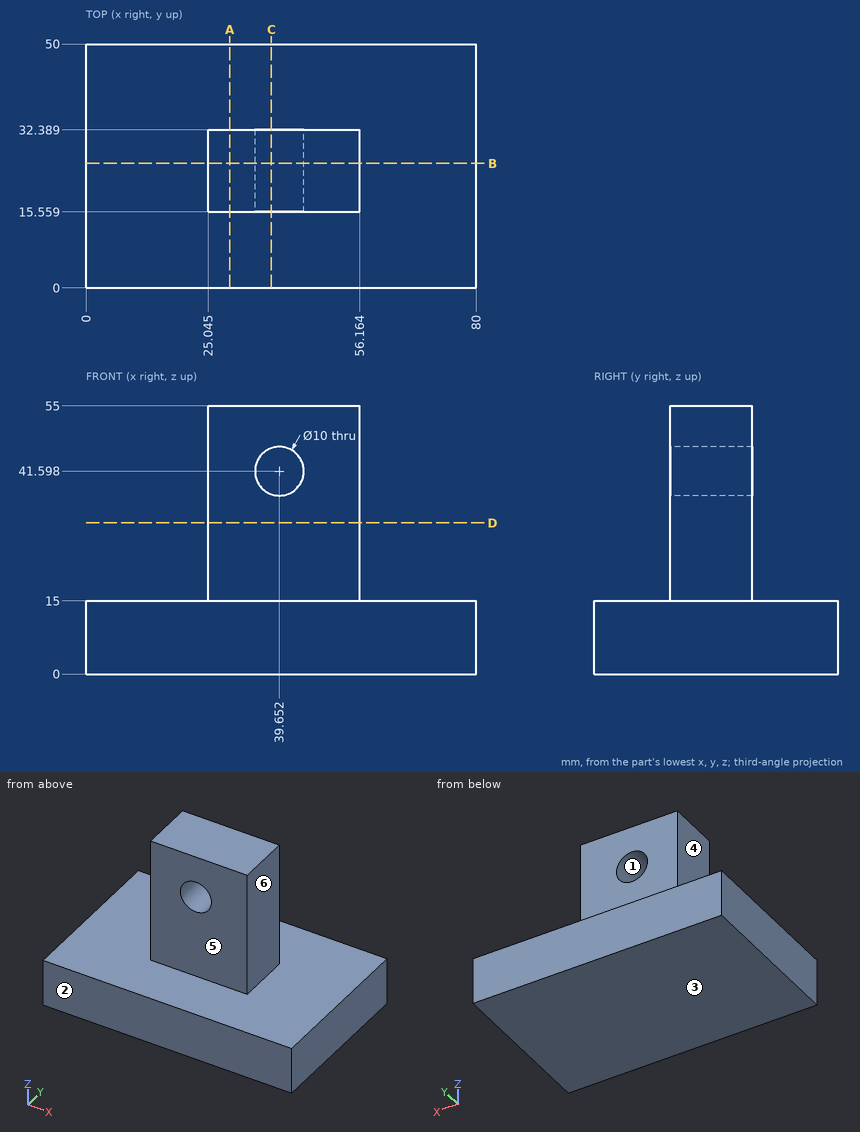
Drawing for the job (mm, zero at the part's lowest x, y, z). A direction names the side the tool comes from. Give positions to 0.01 mm unless a question says otherwise; leave off trailing zeros. Loops run counter-clockwise (first coordinate to the right, second up) from the corner with the lowest first, then second, coordinate; pieces in that order, holes last.
1) Drop flat-ended pins along their axis: P1, Ø1, axis at x = 66.5, y = 8.5, coming from the +Z side; P2, Ø9.5, axis at x = 34, z = 41, coming from the -Y side; P3, Ø6, axis at y = 13.5, z = 44.5, coming from the +X side; P4, Ø12, axis at x = 36, y = 7, coming from the -Z side. Give the stop position or say it passes through.
Values follow:
P1: stops at z = 15
P2: stops at y = 15.56
P3: stops at x = 56.16
P4: stops at z = 0
2) Band-saw the part on D-D on z = 31. List the corners of the cut face in (x, y) (1 decimal), then the cut area to 3 significant figures.
Values follow:
outline: (25, 15.6) - (56.2, 15.6) - (56.2, 32.4) - (25, 32.4) - close
area: 524 mm2
3) Band-saw the part on A-A on x = 29.5. List the corners of the cut face in (y, z), then the cut area to 3 significant figures.
Values follow:
outline: (0, 0) - (50, 0) - (50, 15) - (32.39, 15) - (32.39, 55) - (15.56, 55) - (15.56, 15) - (0, 15) - close
area: 1,420 mm2
4) Two-plate mould, pull along Z, no slides. Class the marked faces 1, 2 and 3: released by +Z, released by -Z, zero draft, split by the parting line, or undercut.
Values follow:
face 1: undercut
face 2: zero draft
face 3: released by -Z
5) Band-saw the part on C-C on x = 38. List the corners of the cut face in (y, z), then the cut area to 3 significant figures.
Values follow:
outline: (0, 0) - (50, 0) - (50, 15) - (32.39, 15) - (32.39, 36.88) - (15.56, 36.88) - (15.56, 15) - (0, 15) - close; (15.56, 46.32) - (32.39, 46.32) - (32.39, 55) - (15.56, 55) - close
area: 1,260 mm2
6) Probe line 1 along Y through (x, z) = (34, 52); line 2 along X through (y, z) = (20, 21) (1 decimal); line 3 along Z through (x, y) = (45.5, 45). List the from-to ranges inside material, lowest first.
Values follow:
line 1: y = 15.56 to 32.39
line 2: x = 25 to 56.2
line 3: z = 0 to 15
7) 3-axis set-ups, long thin cutter, end or side, ignore diameter. For the marked faces 4, 5 and 6: which of +Z, -Z, +X, -X, +Y, -Y reach the whole face in a straight line?
Values follow:
face 4: +Z, -X, +Y, -Y
face 5: +Z, +X, -X, -Y
face 6: +Z, +X, +Y, -Y
8) Band-saw the part on B-B on y = 25.5. List the corners of the cut face in (x, z) (1 decimal), then the cut area to 3 significant figures.
Values follow:
outline: (0, 0) - (80, 0) - (80, 15) - (56.2, 15) - (56.2, 55) - (25, 55) - (25, 15) - (0, 15) - close; hole circle Ø10 at (39.7, 41.6)
area: 2,370 mm2
